Can you work these out from the model? Positions are in its coordinate system, mm. Give positions to 0.01 mm unless a question says otherwise; leave off trailing zeros. Loops run counter-clockwise (first coordinate to the right, second up) from the corner with the lowest first, then second, coordinate; pieces in that order, holes last. Notation, with made-up numbers: (15, 78) -> (59, 78) arc R24 cw to (59, 94) -> close; hole circle Ø2 at (41.5, 16). An arc over 180 degrees is marked (long way). Return JSON: item names as keys, results as strings. Group by question number.
Q1. I need wall thicknesses on line 1 along Z through (x, y) = (0, 4.25); line 2 along X through (y, z) = (5.5, 0.5); line 3 along X through (y, z) = (1.75, -2.5). Which ranges of each line are inside material? Lowest first, please. Write a range as [from, to].
Q2. Suppose I cut it at D-D, the plane z = -48.5. Please give me the cut outline in (x, y), and give its area (3 significant figures).
Q3. Thinking about a two-plate mould opening in Z: for faces 1 (the cylindrical face through (-23.05, 3.13, 1.26)), 2 (the flat face through (-1, 3, 15)), 3 (the flat face through (-27.365, 3.131, -31.482)), 4 (the flat face through (-40, 3, 0)), which applies, pulls with the +Z half, pulls with the -Z half, needs draft (parallel to the pull), parting line crosses it, or undercut?
Q4. Suppose I cut it at C-C, the plane y = 1.75. Please give me the cut outline in (x, z).
Q5. Will these pins go through, and if not, where does the flat tip stop? pin 1 (6 mm diameter, centred on x = 20, z = 0, fed in from +Y); pin 2 (2 mm diameter, centred on y = 3, z = -47, fed in from +X).
Q6. Suppose I cut it at A-A, the plane z = 0. Please give me the cut outline in (x, y), and give its area (3 significant figures).
Q7. Suppose I cut it at B-B, the plane x = 0. Please give me the cut outline in (y, z), and give its area (3 significant figures).
```python
from build123d import *

# Parameters (mm, degrees)
SKETCH1_R            = 14
BOSS_EXTRUDE1_DEPTH  = 6.35
M6_CLEARANCE_HOLE1_D = 6.6


with BuildPart() as part:
    # Sketch1 → Boss-Extrude1 (new body)
    with BuildSketch(Plane(origin=(0, 0, 0), x_dir=(1, 0, 0), z_dir=(0, 1, 0))):
        with BuildLine():
            Line((40, -15), (40, 15))
            Line((40, 15), (15.079194307, 47.509320873))
            ThreePointArc((15.079194307, 47.509320873), (0, 54.95), (-15.079194307, 47.509320873))
            Line((-15.079194307, 47.509320873), (-40, 15))
            Line((-40, 15), (-40, -15))
            Line((-40, -15), (40, -15))
        make_face()
        with Locations((0, 35.95)):
            Circle(SKETCH1_R, mode=Mode.SUBTRACT)
    extrude(amount=BOSS_EXTRUDE1_DEPTH)

    # M6 Clearance Hole1 (through all)
    with Locations(Plane(origin=(0, 6.35, 0), x_dir=(1, 0, 0), z_dir=(0, 1, 0))):
        with Locations((-20, 0), (20, 0)):
            Hole(M6_CLEARANCE_HOLE1_D / 2)


solid = part.part
```
Ans:
{
 "1": {"line 1": "z = [-54.95, -49.95], [-21.95, 15]", "line 2": "x = [-40, -23.26], [-16.74, 16.74], [23.26, 40]", "line 3": "x = [-40, -22.15], [-17.85, 17.85], [22.15, 40]"},
 "2": {"outline": "(-14.27, 0) -> (-6.2, 0) -> (-6.2, 6.35) -> (-14.27, 6.35) -> close; (6.2, 0) -> (14.27, 0) -> (14.27, 6.35) -> (6.2, 6.35) -> close", "area": "102 mm^2"},
 "3": {"face 1": "undercut", "face 2": "pulls with the +Z half", "face 3": "pulls with the -Z half", "face 4": "needs draft"},
 "4": {"outline": "(-40, -15) -> (-15.08, -47.51) arc R19 ccw to (15.08, -47.51) -> (40, -15) -> (40, 15) -> (-40, 15) -> close; hole circle Ø6.6 at (-20, 0); hole circle Ø28 at (0, -35.95); hole circle Ø6.6 at (20, 0)"},
 "5": {"pin 1": "passes through", "pin 2": "stops at x = 16.24"},
 "6": {"outline": "(-40, 0) -> (-23.3, 0) -> (-23.3, 6.35) -> (-40, 6.35) -> close; (-16.7, 0) -> (16.7, 0) -> (16.7, 6.35) -> (-16.7, 6.35) -> close; (23.3, 0) -> (40, 0) -> (40, 6.35) -> (23.3, 6.35) -> close", "area": "424 mm^2"},
 "7": {"outline": "(0, -54.95) -> (6.35, -54.95) -> (6.35, -49.95) -> (0, -49.95) -> close; (0, -21.95) -> (6.35, -21.95) -> (6.35, 15) -> (0, 15) -> close", "area": "266 mm^2"}
}
